Geometry: final body of the model. Coordinates: model frame, mm. Face numbers are marked on the shaded views. A direction names the side the tool comes from. Round coordinates to 2 decimals unless told otherwise and drop trailing zeros. Loops run counter-clockwise (first coordinate to the right, second up) from the corner with the lowest first, then second, coordinate; pieces in that order, holes last. Notation, with made-up numbers: (50.25, -12) - (103.25, -12) arc R15 cw to (103.25, -8) - close; hole circle Ø6 at (-40, 29.25). An arc over 180 degrees is marked (long way). Write item = value, one per line. Start each with the question number.
Item 1: Section C-C (y = 15.5). Return loops of the section in (x, z), plus the area to 3 significant figures.
Item 2: Draft query along X for the marked faces 1, 2, 3 and 4. Return one class per face: pulls with the +X half, pulls with the -X half, needs draft (parallel to the pull), parting line crosses it, or undercut.
Item 3: Section B-B (x = 0). Return loops of the section in (y, z), plus the area to 3 significant figures.
Item 4: Section D-D (z = 34). Return loops of the section in (x, y), plus the area to 3 significant figures.
Item 5: Access query for the marked faces 5 and 6. Directions: +Z, -Z, +X, -X, +Y, -Y. A direction counts if a zero-diameter tool reaches every point of the face in a straight line with its end or side. Return the directions, or none.
Item 6: Line query: line 1 (Z direction, x = 0, y = 64); line 2 (Y direction, x = -20.5, z = -26.5); line 3 (X direction, y = 4.5, z = 34.5). Output: solid intervals per line, ascending. Write a range as from..to.
Item 7: Section A-A (z = 0). Return loops of the section in (x, y), plus the area to 3 significant figures.
from build123d import *

# Parameters (mm, degrees)
F1_DEPTH = 70
F2_R     = 5
F3_W     = 36.3545330494
F3_H     = 25
F4_DEPTH = 102.9998127055
F5_R     = 31.1092179588
F6_DEPTH = 70.001


with BuildPart() as f1:
    # F0 (on Front) → F1 (new body)
    with BuildSketch(Plane.XZ):
        with BuildLine():
            Line((34.6660999328, 54.3679218974), (-71.0870698094, 54.3679218974))
            Line((-71.0870698094, 54.3679218974), (-71.0870698094, -48.6308908081))
            Line((-71.0870698094, -48.6308908081), (34.6660999328, -48.6308908081))
            ThreePointArc((34.6660999328, -48.6308908081), (45.2727016506, -44.2374925259), (49.6660999328, -33.6308908081))
            Line((49.6660999328, -33.6308908081), (49.6660999328, 39.3679218974))
            ThreePointArc((49.6660999328, 39.3679218974), (45.2727016506, 49.9745236152), (34.6660999328, 54.3679218974))
        make_face()
    extrude(amount=-F1_DEPTH)

    # F2
    f2_edges = [f1.edges().sort_by_distance(p)[0] for p in [
        (-71.08707, 0, 2.868516),
        (-71.08707, 70, 2.868516),
    ]]
    fillet(f2_edges, radius=F2_R)

    # F3 (on face) → F4 (cut, through all)
    with BuildSketch(Plane.XY.offset(54.3679218974)):
        with BuildLine():
            Line((34.6660999328, 47.5), (-36.6232544184, 47.5))
            ThreePointArc((-36.6232544184, 47.5), (-49.1232544184, 35), (-36.6232544184, 22.5))
            Line((-36.6232544184, 22.5), (34.6660999328, 22.5))
            Line((34.6660999328, 22.5), (34.6660999328, 47.5))
        make_face()
        with Locations((52.8433664575, 35)):
            Rectangle(F3_W, F3_H)
    extrude(amount=-F4_DEPTH, mode=Mode.SUBTRACT)

    # F5 (on face) → F6 (cut, through all)
    with BuildSketch(Plane.XZ):
        Circle(F5_R)
    extrude(amount=-F6_DEPTH, mode=Mode.SUBTRACT)


solid = f1.part
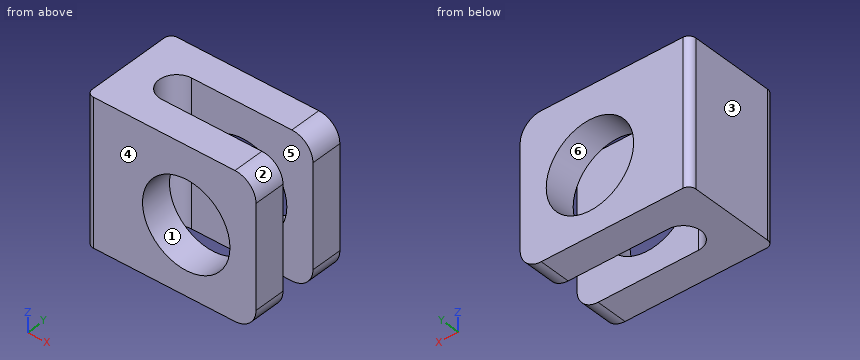
Taken from the geometry:
q1.outline = (-71.09, -48.63) - (34.67, -48.63) arc R15 ccw to (49.67, -33.63) - (49.67, 39.37) arc R15 ccw to (34.67, 54.37) - (-71.09, 54.37) - close; hole circle Ø62.22 at (0, 0)
q1.area = 9,300 mm^2
q2.face_1 = undercut
q2.face_2 = pulls with the +X half
q2.face_3 = pulls with the -X half
q2.face_4 = needs draft
q3.outline = (0, -48.63) - (22.5, -48.63) - (22.5, -31.11) - (0, -31.11) - close; (0, 31.11) - (22.5, 31.11) - (22.5, 54.37) - (0, 54.37) - close; (47.5, -48.63) - (70, -48.63) - (70, -31.11) - (47.5, -31.11) - close; (47.5, 31.11) - (70, 31.11) - (70, 54.37) - (47.5, 54.37) - close
q3.area = 1,840 mm^2
q4.outline = (-71.09, 5) arc R5 ccw to (-66.09, 0) - (49.67, 0) - (49.67, 22.5) - (-36.62, 22.5) arc R12.5 cw to (-36.62, 47.5) - (49.67, 47.5) - (49.67, 70) - (-66.09, 70) arc R5 ccw to (-71.09, 65) - close
q4.area = 6,040 mm^2
q5.face_5 = +Z, -Z, +X
q5.face_6 = +Y, -Y
q6.line_1 = -48.63..-31.11, 31.11..54.37
q6.line_2 = 0..22.5, 47.5..70
q6.line_3 = -71.06..49.67
q7.outline = (-71.09, 5) arc R5 ccw to (-66.09, 0) - (-31.11, 0) - (-31.11, 22.5) - (-36.62, 22.5) arc R12.5 cw to (-36.62, 47.5) - (-31.11, 47.5) - (-31.11, 70) - (-66.09, 70) arc R5 ccw to (-71.09, 65) - close; (31.11, 0) - (49.67, 0) - (49.67, 22.5) - (31.11, 22.5) - close; (31.11, 47.5) - (49.67, 47.5) - (49.67, 70) - (31.11, 70) - close
q7.area = 3,240 mm^2
